```python
from build123d import *

# Parameters (mm, degrees)
EXTRUDE_2_DEPTH     = 14.5
FILLET_2_R          = 6
CUT_EXTRUDE_1_REACH = 62.084
SKETCH_2_R          = 1.75


with BuildPart() as part:
    # 草图1 → 凸台-拉伸2 (new body)
    with BuildSketch(Plane(origin=(0, 0, 0), x_dir=(-1, 0, 0), z_dir=(0, 0, 1))):
        with BuildLine():
            Line((-37.405308562, 24.446583048), (-45.355478911, 16.778806877))
            ThreePointArc((-45.355478911, 16.778806877), (-31.34055986, 20.996004639), (-19.758509765, 12.048444717))
            Line((-19.758509765, 12.048444717), (-8.309528731, 12.048444717))
            ThreePointArc((-8.309528731, 12.048444717), (-6.330928861, 16.982098954), (-3.353982561, 21.385914608))
            ThreePointArc((-3.353982561, 21.385914608), (-10.582575483, 28.195748099), (-13.248153532, 37.762413217))
            ThreePointArc((-13.248153532, 37.762413217), (-22.498153532, 47.012413217), (-31.748153532, 37.762413217))
            ThreePointArc((-31.748153532, 37.762413217), (-33.221077565, 30.528556429), (-37.405308562, 24.446583048))
        make_face()
    extrude(amount=EXTRUDE_2_DEPTH)

    # 圆角2
    fillet_2_edges = [part.edges().sort_by_distance(p)[0] for p in [
        (19.758509765, -12.048444717, 7.25),
    ]]
    fillet(fillet_2_edges, radius=FILLET_2_R)
    fillet_2_2_edges = [part.edges().sort_by_distance(p)[0] for p in [
        (8.309528731, -12.048444717, 7.25),
    ]]
    fillet(fillet_2_2_edges, radius=FILLET_2_R)
    fillet_2_3_edges = [part.edges().sort_by_distance(p)[0] for p in [
        (3.353982561, -21.385914608, 7.25),
    ]]
    fillet(fillet_2_3_edges, radius=FILLET_2_R)
    fillet_2_4_edges = [part.edges().sort_by_distance(p)[0] for p in [
        (45.355478911, -16.778806877, 7.25),
    ]]
    fillet(fillet_2_4_edges, radius=FILLET_2_R)

    # 草图2 → 切除-拉伸1 (cut, up to next)
    with BuildSketch(Plane.XY.offset(14.5), mode=Mode.PRIVATE) as cut_extrude_1_sk1:
        with Locations((22.498153532, -42.762413217)):
            Circle(SKETCH_2_R)
    cut_extrude_1_tool1 = extrude(cut_extrude_1_sk1.sketch, amount=-CUT_EXTRUDE_1_REACH, mode=Mode.PRIVATE) & part.part
    # 草图2 → 切除-拉伸1 (cut, up to next)
    with BuildSketch(Plane.XY.offset(14.5), mode=Mode.PRIVATE) as cut_extrude_1_sk2:
        with Locations((18.168026513, -35.262413217)):
            Circle(SKETCH_2_R)
    cut_extrude_1_tool2 = extrude(cut_extrude_1_sk2.sketch, amount=-CUT_EXTRUDE_1_REACH, mode=Mode.PRIVATE) & part.part
    # 草图2 → 切除-拉伸1 (cut, up to next)
    with BuildSketch(Plane.XY.offset(14.5), mode=Mode.PRIVATE) as cut_extrude_1_sk3:
        with Locations((26.828280551, -35.262413217)):
            Circle(SKETCH_2_R)
    cut_extrude_1_tool3 = extrude(cut_extrude_1_sk3.sketch, amount=-CUT_EXTRUDE_1_REACH, mode=Mode.PRIVATE) & part.part
    # 草图2 → 切除-拉伸1 (cut, up to next)
    with BuildSketch(Plane.XY.offset(14.5), mode=Mode.PRIVATE) as cut_extrude_1_sk4:
        with Locations((28.492231625, -26.496097848)):
            Circle(SKETCH_2_R)
    cut_extrude_1_tool4 = extrude(cut_extrude_1_sk4.sketch, amount=-CUT_EXTRUDE_1_REACH, mode=Mode.PRIVATE) & part.part
    # 草图2 → 切除-拉伸1 (cut, up to next)
    with BuildSketch(Plane.XY.offset(14.5), mode=Mode.PRIVATE) as cut_extrude_1_sk5:
        with Locations((12.488504069, -18.048444717)):
            Circle(SKETCH_2_R)
    cut_extrude_1_tool5 = extrude(cut_extrude_1_sk5.sketch, amount=-CUT_EXTRUDE_1_REACH, mode=Mode.PRIVATE) & part.part
    add(cut_extrude_1_tool1.solids().sort_by_distance((22.498154, -42.762413, 14.5))[0], mode=Mode.SUBTRACT)
    add(cut_extrude_1_tool2.solids().sort_by_distance((18.168027, -35.262413, 14.5))[0], mode=Mode.SUBTRACT)
    add(cut_extrude_1_tool3.solids().sort_by_distance((26.828281, -35.262413, 14.5))[0], mode=Mode.SUBTRACT)
    add(cut_extrude_1_tool4.solids().sort_by_distance((28.492232, -26.496098, 14.5))[0], mode=Mode.SUBTRACT)
    add(cut_extrude_1_tool5.solids().sort_by_distance((12.488504, -18.048445, 14.5))[0], mode=Mode.SUBTRACT)


solid = part.part
```
The listing builds one solid part. Answer for the finished solid, in the listing's coordinates (mm). Round coordinates to 2 decimals unless told otherwise and drop trailing zeros. Order: outer loops, then holes, each group sorted by start corner. A loop starts at its lowest first (then second) coordinate and runs counter-clockwise, first axis right, second up. Notation, with made-up numbers: (6, 26) - (19, 26) arc R20 ccw to (19, 34) - close; hole circle Ø5 at (56, -33.75). An arc over 180 degrees is marked (long way). Put each result on its own line as item: value. Start each with the question number.
(1) Find section B-B (x = 17.5). Give the vertices of the cut face in (y, z).
(2) Find section D-D (x = 8). Give the vertices of the cut face in (y, z).
(3) Given P1, Ø1, axis at y = -16.5, z = 6.5, coming from the -X side; P2, Ø5, axis at y = -16, z = 8.5, coming from the -X side; P3, Ø1, axis at x = 20, y = -26, coming from the -Z side; P4, Ø1, axis at y = -34.5, z = 5.5, coming from the +X side, each flat-ended and moving along its own axis, determine where each tip first touches the part or whether it passes through.
(4) Find section A-A (x = 11.5). Give the vertices of the cut face in (y, z), plus the area to 3 significant figures.
(5) Determine the mould class of faces 1 (the cylindrical face through (6.665, -16.331, 7.148)), 2 (the cylindrical face through (12.109, -19.757, 7.352)), 3 (the cylindrical face through (32.26, -33.44, 7.15)) for opening direction X: released by +X, released by -X, zero draft, split by the parting line, or undercut.
(6) Find section C-C (z = 3.25). State how many separate pieces and enclosed holes the cut face has, plus the area to 3 significant figures.
(7) Straight lines are drawn through the part: probe 1 along Y at (x, z) = (18.5, 8.5); probe 2 along Y at (x, z) = (14, 5.5); probe 3 along X at (y, z) = (-19, 14). For each, find the intervals that lie inside material, in ascending order. Write a range as from..to.
Reply:
1. outline: (-45.55, 0) - (-36.88, 0) - (-36.88, 14.5) - (-45.55, 14.5) - close; (-33.64, 0) - (-12.16, 0) - (-12.16, 14.5) - (-33.64, 14.5) - close
2. outline: (-24.85, 0) - (-14.07, 0) - (-14.07, 14.5) - (-24.85, 14.5) - close
3. P1: x = 6.32
3. P2: x = 5.73
3. P3: z = 0
3. P4: x = 32.13
4. outline: (-29.91, 0) - (-19.49, 0) - (-19.49, 14.5) - (-29.91, 14.5) - close; (-16.6, 0) - (-12.13, 0) - (-12.13, 14.5) - (-16.6, 14.5) - close
4. area: 216 mm^2
5. face 1: released by -X
5. face 2: undercut
5. face 3: released by +X
6. separate pieces: 1
6. enclosed holes: 5
6. area: 613 mm^2
7. probe 1: -46.1..-36.98, -33.54..-12.45
7. probe 2: -41.42..-18.93, -17.17..-12.05
7. probe 3: 5.63..11.02, 13.96..26.05
